Autodesk Fusion 360 part; units mm, degrees
sketch "Skizze1" plane through (0, 0, 0) normal (0, 0, 1) x (1, 0, 0)
  line L0 (0, 0) -> (50, 0)
  line L1 (50, 0) -> (50, 50)
  line L2 (50, 50) -> (0, 50)
  line L3 (0, 50) -> (0, 0)
  line L4 (25, 50) -> (25, -0.5033)
  circle A0 centre (25, 25) radius 11.75
  circle A1 centre (7.5, 17) radius 1.5
  circle A2 centre (42.5, 17) radius 1.5
  circle A3 centre (7.5, 25) radius 4.15
  circle A4 centre (42.5, 25) radius 4.15
  line L5 (9.5, 40.5) -> (40.5, 40.5)
  line L6 (40.5, 40.5) -> (40.5, 9.5)
  line L7 (40.5, 9.5) -> (9.5, 9.5)
  line L8 (9.5, 9.5) -> (9.5, 40.5)
  line L9 (0, 25) -> (50, 25)
  circle A5 centre (9.5, 40.5) radius 3.25
  circle A6 centre (40.5, 40.5) radius 3.25
  circle A7 centre (40.5, 9.5) radius 3.25
  circle A8 centre (9.5, 9.5) radius 3.25
  dimension "d1" = 50
  dimension "d2" = 50
  dimension "d3" = 23.5
  dimension "d4" = 3
  dimension "d5" = 3
  dimension "d6" = 35
  dimension "d7" = 17.5
  dimension "d8" = 8
  dimension "d9" = 8
  dimension "d10" = 25
  dimension "d11" = 8.3
  dimension "d12" = 8.3
  dimension "d13" = 25
  dimension "d14" = 25
  dimension "d15" = 17.5
  dimension "d16" = 17.5
  dimension "d29" = 31
  dimension "d30" = 31
  dimension "d31" = 15.5
  dimension "d32" = 15.5
  dimension "d33" = 6.5
extrude "Extrusion1" add sketch "Skizze1" along normal blind 30 contours L0 L3 L4 A3 L7 L8 L9 A8 | L0 L1 L4 A4 L6 L7 L9 A7 | L2 L3 L4 A3 L5 L8 L9 A5 | L4 A0 A3 L7 L8 L9 A8 | L4 A0 A4 L6 L7 L9 A7 | A3 L8 L9 | A3 L8 L9 | L1 L2 L4 A4 L5 L6 L9 A6 | L4 A0 A3 L5 L8 L9 A5 | A3 L8 L9 | A3 L8 L9 | A4 L6 L9 | A4 L6 L9 | L4 A0 A4 L5 L6 L9 A6 | A4 L6 L9 | A4 L6 L9 | A1 | A2
extrude "Extrusion2" cut sketch "Skizze1" along normal blind 20 contours A3 L8 L9 | A3 L8 L9 | A3 L8 L9 | A3 L8 L9 | A4 L6 L9 | A4 L6 L9 | A4 L6 L9 | A4 L6 L9
sketch "Skizze2" plane through (0, 0, 30) normal (0, 0, 1) x (-1, 0, 0)
  circle A0 centre (-25, -25) radius 11.75
  line L0 (0, -50) -> (0, 0)
  line L1 (0, 0) -> (-50, 0)
  line L2 (-50, 0) -> (-50, -50)
  line L3 (-50, -50) -> (0, -50)
  circle A1 centre (-7.5, -17) radius 1.5
  circle A2 centre (-42.5, -17) radius 1.5
  circle A3 centre (-40.5, -40.5) radius 3.25
  circle A4 centre (-9.5, -9.5) radius 3.25
  circle A5 centre (-40.5, -9.5) radius 3.25
  circle A6 centre (-9.5, -40.5) radius 3.25
  circle A7 centre (-9.5, -40.5) radius 3.25
  circle A8 centre (-40.5, -40.5) radius 3.25
  circle A9 centre (-40.5, -9.5) radius 3.25
  circle A10 centre (-9.5, -9.5) radius 3.25
  circle A11 centre (-9.5, -40.5) radius 1.75
  circle A12 centre (-40.5, -40.5) radius 1.75
  circle A13 centre (-40.5, -9.5) radius 1.75
  circle A14 centre (-9.5, -9.5) radius 1.75
  point P0 (-25, -25)
  dimension "d21" = 3
  dimension "d22" = 3
  dimension "d23" = 17.5
  dimension "d24" = 17.5
  dimension "d25" = 8
  dimension "d26" = 8
  dimension "d34" = 6.5
  dimension "d35" = 3.5
extrude "Extrusion3" cut sketch "Skizze2" against normal blind 15 contours A1 | A2
extrude "Extrusion4" add sketch "Skizze2" against normal blind 5 contours A3 A8 | A4 A10 | A5 A9 | A6 A7
fillet "Abrundung1" radius 10 4 edges at (50, 50, 15) (50, 0, 15) (0, 0, 15) (0, 50, 15)
equation "d7 = ( 35 / 2 ) * 1 mm"
equation "d31 = ( 31 / 2 ) * 1 mm"
equation "d32 = ( 31 / 2 ) * 1 mm"
The model under review builds one solid part; all positions refer to its coordinate system, in mm. A direction names the side the tool comes from. Give positions to 0.01 mm unless a question says otherwise; leave off trailing zeros. Order: outer loops, then holes, each group sorted by start corner. A loop starts at its lowest first (then second) coordinate and runs counter-clockwise, first axis right, second up. Notation, with made-up numbers: M -36.75,79 L -6.75,79 A25 ccw -6.75,95 Z; hole C 40,6 d1. An arc over 180 degrees is marked long. Answer in a Markdown table with one row per item. Add a question column.
1. Mouldability with a two-part tool opening along X and no side actions: class faces 4 (the cylindrical face through (44, 17, 23)), 5 (the cylindrical face through (2.85, 3.01, 15.21)), 6 (the flat face through (25, 0, 15)) as released by +X, released by -X, zero draft, split by the parting line, or undercut.
2. Add section C-C on z = 19. Count the separate pieces of the cut face and the enclosed holes in it, plus the area to 3 significant figures.
3. Add section D-D on z = 26. State the section outline as (x, y) points.
4. Add section A-A on y = 17. State the section outline as (x, z) points, plus the area to 3 significant figures.
5. Add section B-B on x = 24. State the section outline as (y, z) points.
6. Machinability: for faces 1 (the flat face through (8, 17, 15)), 2 (the flat face through (39, 11, 25)), 3 (the cylindrical face through (38.831, 8.974, 27.535)), which of the approach directions +Z, -Z, +X, -X, +Y, -Y give a long, thin tool a straight path to every point of the face, cutting with its end or side? Answer none if there is none.
7. To check wall thickness, follow line 1 along X through (y, z) = (40.5, 27.65); line 2 along X through (y, z) = (25, 8.5). State the ranges of each line that lie inside material, in increasing order.
8. For pin 1 Ø1.5 at (y, z) = (45, 26.5) entering from -X; pin 2 Ø6 at (x, y) = (30, 44) entering from -Z; pin 3 Ø2 at (x, y) = (40.5, 9.5) entering from -Z; pin 4 Ø1.5 at (x, y) = (42.5, 17.5) entering from +Z, all flat-tipped, find the tip position at first contact; note any pin that passes through.
The answers:
| question | item | result |
|---|---|---|
| 1 | face 4 | undercut |
| 1 | face 5 | released by -X |
| 1 | face 6 | zero draft |
| 2 | separate pieces | 1 |
| 2 | enclosed holes | 9 |
| 2 | area | 1,730 mm2 |
| 3 | outline | M 0,10 A10 ccw 10,0 L 40,0 A10 ccw 50,10 L 50,40 A10 ccw 40,50 L 10,50 A10 ccw 0,40 Z; hole C 7.5,17 d3; hole C 9.5,9.5 d3.5; hole C 9.5,40.5 d3.5; hole C 25,25 d23.5; hole C 40.5,9.5 d3.5; hole C 40.5,40.5 d3.5; hole C 42.5,17 d3 |
| 4 | outline | M 0,0 L 16.39,0 L 16.39,30 L 9,30 L 9,15 L 6,15 L 6,30 L 0,30 Z; M 33.61,0 L 50,0 L 50,30 L 44,30 L 44,15 L 41,15 L 41,30 L 33.61,30 Z |
| 4 | area | 894 mm2 |
| 5 | outline | M 0,0 L 13.29,0 L 13.29,30 L 0,30 Z; M 36.71,0 L 50,0 L 50,30 L 36.71,30 Z |
| 6 | face 1 | +Z |
| 6 | face 2 | -Z |
| 6 | face 3 | +Z, -Z |
| 7 | line 1 | 0.01 to 7.75, 11.25 to 38.75, 42.25 to 49.99 |
| 7 | line 2 | 0 to 3.35, 11.65 to 13.25, 36.75 to 38.35, 46.65 to 50 |
| 8 | pin 1 | x = 0.95 |
| 8 | pin 2 | z = 0 |
| 8 | pin 3 | through |
| 8 | pin 4 | z = 15 |
